```python
from build123d import *

# Parameters (mm, degrees)
F0_W            = 100
F0_H            = 80
F1_DEPTH        = 3
F4_DEPTH        = 15
F6_DEPTH        = 15.001
F3_W            = 25.5
F3_H            = 30
F7_DEPTH        = 28
F8_W            = 50
F8_H            = 50
F9_DEPTH        = 6
F10_D           = 4
F10_CBORE_D     = 6.5
F10_CBORE_DEPTH = 3
F11_D           = 3
F11_CBORE_D     = 6.5
F11_CBORE_DEPTH = 3
F12_D           = 3
F12_CBORE_D     = 5
F12_CBORE_DEPTH = 3


with BuildPart() as f1:
    # F0 (on Top) → F1 (new body)
    with BuildSketch(Plane.XY):
        Rectangle(F0_W, F0_H)
    extrude(amount=F1_DEPTH)

    # F2 (on face) → F4 (join)
    with BuildSketch(Plane(origin=(0, 0, 0), x_dir=(1, 0, 0), z_dir=(0, 0, -1))):
        with BuildLine():
            Line((-50, 40), (-16.5, 40))
            ThreePointArc((-16.5, 40), (-40.6899033384, 57.6032667423), (-50, 29.1717960861))
            Line((-50, 29.1717960861), (-50, 40))
        make_face()
        with BuildLine():
            ThreePointArc((-50, 29.1717960861), (-29.3100966616, 22.3967332577), (-16.5, 40))
            Line((-16.5, 40), (-50, 40))
            Line((-50, 40), (-50, 29.1717960861))
        make_face()
        with BuildLine():
            Line((50, 40), (16.5, 40))
            ThreePointArc((16.5, 40), (29.3100966616, 22.3967332577), (50, 29.1717960861))
            Line((50, 29.1717960861), (50, 40))
        make_face()
        with BuildLine():
            ThreePointArc((53.5, 40), (35, 58.5), (16.5, 40))
            Line((16.5, 40), (50, 40))
            Line((50, 40), (50, 29.1717960861))
            ThreePointArc((50, 29.1717960861), (52.6032667423, 34.3100966616), (53.5, 40))
        make_face()
    extrude(amount=-F4_DEPTH)

    # F5 (on face) → F6 (cut, through all)
    with BuildSketch(Plane.XY.offset(15)):
        with BuildLine():
            Line((-27, -56.6808273176), (-27, -40))
            ThreePointArc((-27, -40), (-31.9385325411, -32.6089637399), (-40.6568542495, -34.3431457505))
            Line((-40.6568542495, -34.3431457505), (-52.4519803616, -46.1382718626))
            ThreePointArc((-52.4519803616, -46.1382718626), (-42.0796434988, -57.0917713515), (-27, -56.6808273176))
        make_face()
        with BuildLine():
            ThreePointArc((40.6568542495, -34.3431457505), (31.9385325411, -32.6089637399), (27, -40))
            Line((27, -40), (27, -56.6808273176))
            ThreePointArc((27, -56.6808273176), (42.0796434988, -57.0917713515), (52.4519803616, -46.1382718626))
            Line((52.4519803616, -46.1382718626), (40.6568542495, -34.3431457505))
        make_face()
    extrude(amount=-F6_DEPTH, mode=Mode.SUBTRACT)

    # F3 (on Top) → F7 (join)
    with BuildSketch(Plane.XY):
        with Locations((-37.25, 12)):
            Rectangle(F3_W, F3_H)
        with Locations((37.25, 12)):
            Rectangle(F3_W, F3_H)
    extrude(amount=F7_DEPTH)

    # F8 (on Top) → F9 (join)
    with BuildSketch(Plane.XY):
        with Locations((0, 12)):
            Rectangle(F8_W, F8_H)
    extrude(amount=F9_DEPTH)

    # F10 (through all)
    with Locations(Plane(origin=(0, 0, 0), x_dir=(1, 0, 0), z_dir=(0, 0, -1))):
        with Locations((-20.25, 8), (20.25, 8), (-20.25, -32), (20.25, -32)):
            CounterBoreHole(F10_D / 2, F10_CBORE_D / 2, F10_CBORE_DEPTH)

    # F11 (through all)
    with Locations(Plane(origin=(0, 0, 0), x_dir=(1, 0, 0), z_dir=(0, 0, -1))):
        with Locations((-46.2583302492, 33.5), (-46.2583302492, 46.5), (-23.7416697508, 46.5), (-23.7416697508, 33.5), (-35, 27), (23.7416697508, 46.5), (46.2583302492, 46.5), (46.2583302492, 33.5), (35, 27), (23.7416697508, 33.5)):
            CounterBoreHole(F11_D / 2, F11_CBORE_D / 2, F11_CBORE_DEPTH)

    # F12 (through all)
    with Locations(Plane(origin=(0, 0, 0), x_dir=(1, 0, 0), z_dir=(0, 0, -1))):
        with Locations((-28.5, -22.25), (-28.5, -1.75), (28.5, -22.25), (28.5, -1.75)):
            CounterBoreHole(F12_D / 2, F12_CBORE_D / 2, F12_CBORE_DEPTH)


solid = f1.part
```
Could you check a few things on this model? Use its own coordinates, in mm. A direction names the side the tool comes from. Coordinates: 2 decimals unless noted, no trailing zeros. Write each loop counter-clockwise with the first axis right and the second up, starting at its lowest first coordinate (ties: lowest second). Pieces come first, ordered by that corner, then holes. Notation, with made-up numbers: (78, -16) -> (116, -16) arc R18 cw to (116, 11) -> close; hole circle Ø11 at (37, 34). An arc over 180 degrees is marked (long way). Write item = value, one per line. Start each with the question number.
(1) I want a section at C-C (z = 17). Please give me the cut outline in (x, y).
(2) I want a section at B-B (x = 35). Please give me the cut outline in (y, z), plus the area to 3 significant figures.
(3) I want a section at D-D (z = 4.25). Give the number of separate pieces and of enclosed holes in the cut face, plus the area to 3 significant figures.
(4) I want a section at A-A (y = -8). Please give me the cut outline in (x, z).
(5) We'd pull the mould along X, two halves only. Please class faces 5 (the face through (34.7, -31.5, 15)), 6 (the face through (23, -45, 3)), 7 (the face through (-25, 32, 4)): released by +X, released by -X, zero draft, split by the parting line, or undercut.
(6) Will these pins go through, and if not, where does the flat tip stop? pin 1 (2 mm diameter, centred on y = 14, z = 3, fed in from +X); pin 2 (7 mm diameter, centred on x = 19, y = -9, fed in from -Z); pin 3 (4 mm diameter, centred on x = -23.74, y = -46.5, fed in from +Z); pin 4 (2 mm diameter, centred on y = -31, z = 8.5, fed in from +X).
(7) Which directions (+Z, -Z, +X, -X, +Y, -Y) give clear straight access to the entire face, cutting with the end or side of a thin tool? Please do faces 1 (the face through (-25, -8, 4)), 2 (the face through (-22.242, -43.617, 1.479)), 3 (the face through (-27, -48, 8)), 4 (the face through (0, 37, 4)).
(8) I need wall thicknesses on line 1 (Y direction, x = -35, z = 12); line 2 (Y direction, x = 28.5, z = 17); line 3 (X direction, y = 10, z = 9.5). Which ranges of each line are inside material? Lowest first, please. Write a range as [from, to].
Result set:
q1.outline = (-50, -3) -> (-24.5, -3) -> (-24.5, 27) -> (-50, 27) -> close; (24.5, -3) -> (50, -3) -> (50, 27) -> (24.5, 27) -> close; hole circle Ø3 at (-28.5, 1.75); hole circle Ø3 at (-28.5, 22.25); hole circle Ø3 at (28.5, 1.75); hole circle Ø3 at (28.5, 22.25)
q2.outline = (-32, 0) -> (-30.25, 0) -> (-30.25, 3) -> (-28.5, 3) -> (-28.5, 15) -> (-32, 15) -> close; (-25.5, 3) -> (-23.75, 3) -> (-23.75, 0) -> (40, 0) -> (40, 3) -> (27, 3) -> (27, 28) -> (-3, 28) -> (-3, 3) -> (-21.5, 3) -> (-21.5, 15) -> (-25.5, 15) -> close
q2.area = 1,040 mm2
q3.separate_pieces = 3
q3.enclosed_holes = 16
q3.area = 5,020 mm2
q4.outline = (-50, 0) -> (-23.5, 0) -> (-23.5, 3) -> (-22.25, 3) -> (-22.25, 6) -> (-25, 6) -> (-25, 3) -> (-50, 3) -> close; (-18.25, 3) -> (-17, 3) -> (-17, 0) -> (17, 0) -> (17, 3) -> (18.25, 3) -> (18.25, 6) -> (-18.25, 6) -> close; (22.25, 3) -> (23.5, 3) -> (23.5, 0) -> (50, 0) -> (50, 3) -> (25, 3) -> (25, 6) -> (22.25, 6) -> close
q5.face_5 = zero draft
q5.face_6 = undercut
q5.face_7 = released by -X
q6.pin_1 = 50
q6.pin_2 = 0
q6.pin_3 = 15
q6.pin_4 = 51.68
q7.face_1 = +Z, -X
q7.face_2 = -Z
q7.face_3 = +Z, -Z, -Y
q7.face_4 = +Z, +X, -X, +Y
q8.line_1 = [-32, -28.5], [-25.5, -21.5], [-3, 27]
q8.line_2 = [-3, 0.25], [3.25, 20.75], [23.75, 27]
q8.line_3 = [-50, -24.5], [24.5, 50]
